```python
from build123d import *

# Parameters (mm, degrees)
SKETCH1_R            = 15.875
SKETCH1_R_2          = 12.7
BOSS_EXTRUDE1_DEPTH  = 15
BOSS_EXTRUDE2_DEPTH  = 10
CUT_EXTRUDE1_DEPTH   = 5
M5_CLEARANCE_HOLE1_D = 5.5


with BuildPart() as part:
    # Sketch1 → Boss-Extrude1 (new, symmetric)
    with BuildSketch(Plane.XY):
        Circle(SKETCH1_R)
        Circle(SKETCH1_R_2, mode=Mode.SUBTRACT)
    extrude(amount=BOSS_EXTRUDE1_DEPTH, both=True)

    # Sketch3 → Boss-Extrude2 (add, symmetric)
    with BuildSketch(Plane.XY):
        with BuildLine():
            Line((-11.276400848, 11.174005948), (-11.276400848, 26.174005948))
            ThreePointArc((-11.276400848, 26.174005948), (-8.34746866, 33.245073759), (-1.276400848, 36.174005948))
            Line((-1.276400848, 36.174005948), (1.276400848, 36.174005948))
            ThreePointArc((1.276400848, 36.174005948), (8.34746866, 33.245073759), (11.276400848, 26.174005948))
            Line((11.276400848, 26.174005948), (11.276400848, 11.174005948))
            ThreePointArc((11.276400848, 11.174005948), (0, 15.875), (-11.276400848, 11.174005948))
        make_face()
    extrude(amount=BOSS_EXTRUDE2_DEPTH, both=True)

    # Sketch3<2> → Cut-Extrude1 (cut, symmetric)
    with BuildSketch(Plane.XY):
        with BuildLine():
            Line((-11.276400848, 11.174005948), (-11.276400848, 26.174005948))
            ThreePointArc((-11.276400848, 26.174005948), (-8.34746866, 33.245073759), (-1.276400848, 36.174005948))
            Line((-1.276400848, 36.174005948), (1.276400848, 36.174005948))
            ThreePointArc((1.276400848, 36.174005948), (8.34746866, 33.245073759), (11.276400848, 26.174005948))
            Line((11.276400848, 26.174005948), (11.276400848, 11.174005948))
            ThreePointArc((11.276400848, 11.174005948), (0, 15.875), (-11.276400848, 11.174005948))
        make_face()
    extrude(amount=CUT_EXTRUDE1_DEPTH, both=True, mode=Mode.SUBTRACT)

    # M5 Clearance Hole1 (through all)
    with Locations(Plane.XY.offset(10)):
        with Locations((0, 26.174005948)):
            Hole(M5_CLEARANCE_HOLE1_D / 2)


solid = part.part
```
Geometry check sheet. Reference: the model listing, model coordinates, mm. A direction names the side the tool comes from. Coordinates: 2 decimals unless noted, no trailing zeros. Loops run counter-clockwise (first coordinate to the right, second up) from the corner with the lowest first, then second, coordinate; pieces in that order, holes last. Notation, with made-up numbers: (75.5, 44.5) - (109.5, 44.5) arc R12 cw to (109.5, 62.5) - close; hole circle Ø3 at (77.25, -20.5). An arc over 180 degrees is marked (long way). One line per item, written item: value. Start each with the question number.
(1) Tool access check on faces 4 (the flat face through (11.276, 19, 8)), 5 (the cylindrical face through (-2.75, -12.4, -0.21)), 6 (the flat face through (-11.276, 19, 8)). Record the directions out of +Z, -Z, +X, -X, +Y, -Y that give a thin tool (end or side, any length) a straight path to the whole face; none if there is none.
(2) Depth check by flat-ended pin: P1, Ø4, axis at x = 9.5, y = 27, coming from the -Z side; P2, Ø1, axis at y = -6, z = -7, coming from the +X side; P3, Ø1, axis at x = 5.5, z = 8, coming from the +Y side. Enter the tip coordinate at first touch or a pass-through.
(3) Material ranges on line 1 (Y direction, x = 0, z = -6.1) (3 decimals); line 2 (Z direction, x = 3.5, y = 17); line 3 (Y direction, x = -5, z = 10.75), recorded low to high. Write a range as [from, to].
(4) Cross-section at D-D on x = -4. Enter the section's corners in (y, z).
(5) Cross-section at A-A on x = 0. Enter the section's corners in (y, z) (3 decimals), plus the area to 3 significant figures.
(6) Mould release check, pull along X, two halves, no side actions. Record for faces 1 (the flat face through (11.276, 19, -7)), 2 (the cylindrical face through (0.36, 28.9, 7.47)), 3 (the flat face through (-7, 11, -15)): released by +X, released by -X, zero draft, split by the parting line, or undercut.
(7) Cross-section at C-C on z = 6. Enter the section's corners in (x, y) (3 decimals).
(8) Cross-section at B-B on y = 0. Enter the section's corners in (x, z) (3 decimals).
Results below:
1. face 4: +Z, -Z, +X, +Y
1. face 5: +Z, -Z
1. face 6: +Z, -Z, -X, +Y
2. P1: stops at z = -10
2. P2: stops at x = 14.89
2. P3: stops at y = 35.45
3. line 1: y = [-15.875, -12.7], [12.7, 23.424], [28.924, 36.174]
3. line 2: z = [-10, -5], [5, 10]
3. line 3: y = [-15.07, -11.67], [11.67, 15.07]
4. outline: (-15.36, -15) - (-12.05, -15) - (-12.05, 15) - (-15.36, 15) - close; (12.05, -15) - (15.36, -15) - (15.36, -10) - (35.8, -10) - (35.8, -5) - (15.36, -5) - (15.36, 5) - (35.8, 5) - (35.8, 10) - (15.36, 10) - (15.36, 15) - (12.05, 15) - close
5. outline: (-15.875, -15) - (-12.7, -15) - (-12.7, 15) - (-15.875, 15) - close; (12.7, -15) - (15.875, -15) - (15.875, -10) - (23.424, -10) - (23.424, -5) - (15.875, -5) - (15.875, 5) - (23.424, 5) - (23.424, 10) - (15.875, 10) - (15.875, 15) - (12.7, 15) - close; (28.924, -10) - (36.174, -10) - (36.174, -5) - (28.924, -5) - close; (28.924, 5) - (36.174, 5) - (36.174, 10) - (28.924, 10) - close
5. area: 338 mm2
6. face 1: released by +X
6. face 2: undercut
6. face 3: zero draft
7. outline: (-11.276, 11.174) arc R15.875 ccw (long way) to (11.276, 11.174) - (11.276, 26.174) arc R10 ccw to (1.276, 36.174) - (-1.276, 36.174) arc R10 ccw to (-11.276, 26.174) - close; hole circle Ø25.4 at (0, 0); hole circle Ø5.5 at (0, 26.174)
8. outline: (-15.875, -15) - (-12.7, -15) - (-12.7, 15) - (-15.875, 15) - close; (12.7, -15) - (15.875, -15) - (15.875, 15) - (12.7, 15) - close
